```python
from build123d import *

# Parameters (mm, degrees)
BOSS_EXTRUDE1_DEPTH = 70
SKETCH4_R           = 17.5
CUT_EXTRUDE3_DEPTH  = 137
SKETCH6_W           = 25
SKETCH6_H           = 50
CUT_EXTRUDE4_DEPTH  = 137
SKETCH7_W           = 25
SKETCH7_H           = 50
CUT_EXTRUDE5_DEPTH  = 137
CUT_EXTRUDE6_DEPTH  = 137


with BuildPart() as part:
    # Sketch3 → Boss-Extrude1 (new body)
    with BuildSketch(Plane.XY):
        Polygon((24.962893573, 73.456383547), (24.962893573, -61.543616453), (-5.037106427, -61.543616453), (-5.037106427, 13.456383547), (-35.037106427, 13.456383547), (-35.037106427, -61.543616453), (-65.037106427, -61.543616453), (-65.037106427, 48.456383547), (-25.037106427, 73.456383547), align=None)
    extrude(amount=BOSS_EXTRUDE1_DEPTH)

    # Sketch4 → Cut-Extrude3 (cut)
    with BuildSketch(Plane.ZY.offset(65.037106427)):
        with Locations((35, -26.543616453)):
            Circle(SKETCH4_R)
    extrude(amount=-CUT_EXTRUDE3_DEPTH, mode=Mode.SUBTRACT)

    # Sketch6 → Cut-Extrude4 (cut)
    with BuildSketch(Plane(origin=(24.962893573, 0, 0), x_dir=(0, 0, -1), z_dir=(1, 0, 0))):
        with Locations((-57.5, 48.456383547)):
            Rectangle(SKETCH6_W, SKETCH6_H)
    extrude(amount=-CUT_EXTRUDE4_DEPTH, mode=Mode.SUBTRACT)

    # Sketch7 → Cut-Extrude5 (cut)
    with BuildSketch(Plane(origin=(24.962893573, 0, 0), x_dir=(0, 0, -1), z_dir=(1, 0, 0))):
        with Locations((-12.5, 48.456383547)):
            Rectangle(SKETCH7_W, SKETCH7_H)
    extrude(amount=-CUT_EXTRUDE5_DEPTH, mode=Mode.SUBTRACT)

    # Sketch8 → Cut-Extrude6 (cut)
    with BuildSketch(Plane.ZY.offset(65.037106427)):
        with BuildLine():
            ThreePointArc((35, -61.543616453), (10.251262658, -51.292353794), (0, -26.543616453))
            Line((0, -26.543616453), (0, -61.543616453))
            Line((0, -61.543616453), (35, -61.543616453))
        make_face()
        with BuildLine():
            Line((70, -61.543616453), (70, -26.543616453))
            ThreePointArc((70, -26.543616453), (59.748737342, -51.292353794), (35, -61.543616453))
            Line((35, -61.543616453), (70, -61.543616453))
        make_face()
    extrude(amount=-CUT_EXTRUDE6_DEPTH, mode=Mode.SUBTRACT)


solid = part.part
```
Could you check a few things on this model? Use its own coordinates, in mm. A direction names the side the tool comes from. Round coordinates to 2 decimals unless told otherwise and drop trailing zeros. Loops run counter-clockwise (first coordinate to the right, second up) from the corner with the lowest first, then second, coordinate; pieces in that order, holes last. Notation, with made-up numbers: M 74,6 L 131,6 A12 ccw 131,25 Z; hole C -38.75,0 d4. An arc over 180 degrees is marked long. Answer as CSV lines item,"result".
1) We'd pull the mould along Z, two halves only. Please class faces 1 (the flat face through (-65.037, -7, 35)), 2 (the cylindrical face through (-50.247, -42.069, 43.075)), 3 (the cylindrical face through (9.753, -42.069, 43.075)), 4 (the flat face through (-19, 15, 70)): released by +Z, released by -Z, zero draft, split by the parting line, or undercut.
From the geometry:
face 1,"zero draft"
face 2,"undercut"
face 3,"undercut"
face 4,"released by +Z"
2) Imagine slicing it at A-A on y = -40.5. List the corners of the cut face in (x, z) for me.
From the geometry:
outline,"M -65.04,2.9 L -35.04,2.9 L -35.04,24.44 L -65.04,24.44 Z; M -65.04,45.56 L -35.04,45.56 L -35.04,67.1 L -65.04,67.1 Z; M -5.04,2.9 L 24.96,2.9 L 24.96,24.44 L -5.04,24.44 Z; M -5.04,45.56 L 24.96,45.56 L 24.96,67.1 L -5.04,67.1 Z"
3) Which directions (+Z, -Z, +X, -X, +Y, -Y) give clear straight access to the entire face, cutting with the end or side of a thin tool? Please do faces 5 (the flat face through (-19, 23.456, 58)), 6 (the flat face through (-19, 48, 25)), 7 (the flat face through (-35.037, -7, 35)), 8 (the flat face through (-45.32, 60.78, 34.86)), 9 (the flat face through (24.963, 7, 35)).
From the geometry:
face 5,"+Z, +X, -X, +Y"
face 6,"-Z, +X, -X, +Y"
face 7,"+Z, -Z, -Y"
face 8,"+Z, -Z, -X, +Y"
face 9,"+Z, -Z, +X, +Y, -Y"
4) Imagine slicing it at B-B on z = 42.5. List the corners of the cut face in (x, y) for me (3 decimals).
From the geometry:
outline,"M -65.037,-60.731 L -35.037,-60.731 L -35.037,-42.355 L -65.037,-42.355 Z; M -65.037,-10.732 L -35.037,-10.732 L -35.037,13.456 L -5.037,13.456 L -5.037,-10.732 L 24.963,-10.732 L 24.963,73.456 L -25.037,73.456 L -65.037,48.456 Z; M -5.037,-60.731 L 24.963,-60.731 L 24.963,-42.355 L -5.037,-42.355 Z"
5) For pin 1 Ø20 at (x, z) = (-28.5, 15.5) entering from +Y; pin 2 Ø15 at (x, z) = (-23.5, 37) entering from -Y; pin 3 Ø25 at (x, y) = (-30.5, 43) entering from +Z; pin 4 Ø12 at (x, y) = (-50.5, -4.5) entering from -Z, each with a flat end and sliding along its axis, tell me the tip position at first contact or that it passes through.
From the geometry:
pin 1,"y = 73.24"
pin 2,"y = 13.46"
pin 3,"z = 45"
pin 4,"z = 0"
6) If I drill on probe 1 along X at (y, z) = (-2, 4); probe 2 along Y at (x, z) = (14.25, 35); probe 3 along Z at (x, y) = (4, 60), over which ranges is the centre line in solid material (lowest first)?
From the geometry:
probe 1,"-65.04 to -35.04, -5.04 to 24.96"
probe 2,"-61.54 to -44.04, -9.04 to 73.46"
probe 3,"25 to 45"
7) Imagine slicing it at D-D on x = -55. List the corners of the cut face in (y, z) for me, and give its area (3 significant figures).
From the geometry:
outline,"M -26.54,0 L 23.46,0 L 23.46,25 L 54.73,25 L 54.73,45 L 23.46,45 L 23.46,70 L -26.54,70 A35 ccw Z; hole C -26.54,35 d35"
area,"5,090 mm^2"
8) Imagine slicing it at C-C on z = 57.5. List the corners of the cut face in (x, y) for me.
From the geometry:
outline,"M -65.04,-53.35 L -35.04,-53.35 L -35.04,13.46 L -5.04,13.46 L -5.04,-53.35 L 24.96,-53.35 L 24.96,23.46 L -65.04,23.46 Z"
